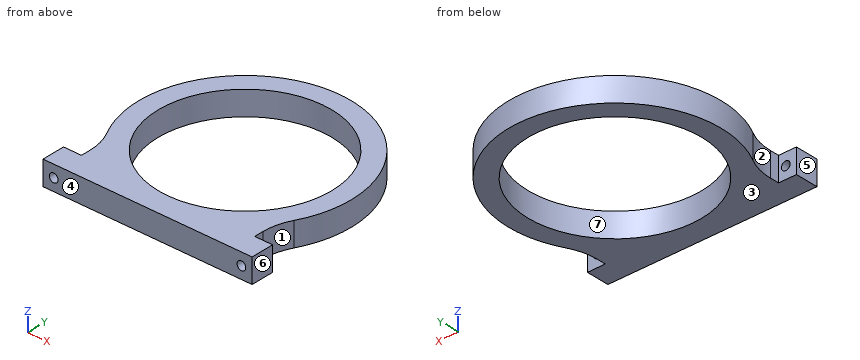
Autodesk Inventor part; units mm, degrees
ref_plane "YZ Plane" through (0, 0, 0) normal (1, 0, 0) x (0, 1, 0)
ref_plane "XZ Plane" through (0, 0, 0) normal (0, 1, 0) x (-1, 0, 0)
ref_plane "XY Plane" through (0, 0, 0) normal (0, 0, 1) x (1, 0, 0)
sketch "Sketch1" plane through (0, 0, 0) normal (0, 0, 1) x (1, 0, 0)
  line L0 (0, 0) -> (72.4, 0)
  line L1 (72.4, 0) -> (72.4, 8)
  line L2 (72.4, 8) -> (0, 8)
  line L3 (0, 8) -> (0, 0)
  line L4 (36.2, 8) -> (36.2, 38) construction
  circle A0 centre (36.2, 38) radius 30
  circle A1 centre (36.2, 38) radius 36.75
  line L5 (6.2, 8) -> (6.2, 16.7735)
  line L6 (66.2, 8) -> (66.2, 16.7735)
  dimension "d0" = 72.4
  dimension "d1" = 8
  dimension "d2" = 30
  dimension "d3" = 60
  dimension "d4" = 73.5
extrude "Extrusion1" add sketch "Sketch1" along normal blind 8.4
fillet "Fillet1" radius 20 2 edges at (66.2, 16.7735, 4.2) (6.2, 16.7735, 4.2)
sketch "Sketch2" plane through (0, 0, 0) normal (0, -1, 0) x (1, 0, 0)
  line L0 (72.4, 0) -> (72.4, 8.4)
  line L1 (0, 0) -> (0, 8.4) construction
  line L2 (0, 4.2) -> (3.7, 4.2) construction
  circle A0 centre (3.7, 4.2) radius 1.5
  line L3 (72.4, 4.2) -> (68.7, 4.2) construction
  circle A1 centre (68.7, 4.2) radius 1.5
  dimension "d8" = 3.7
  dimension "d9" = 3
  dimension "d10" = 3.7
  dimension "d11" = 3
extrude "Extrusion2" cut sketch "Sketch2" against normal up to surface (8 mm away)
properties part number "reservoir pump combo mount"
Can you work these out from the model? Positions are in its coordinate system, mm. Face numbers are marked on the shaded views. A direction names the side the tool comes from. Coordinates: 2 decimals unless noted, no trailing zeros. Loops run counter-clockwise (first coordinate to the right, second up) from the corner with the lowest first, then second, coordinate; pieces in that order, holes last. Notation, with made-up numbers: M 83.25,-28 L 99.25,-28 A29 ccw 99.25,-1 Z; hole C -27.75,33.5 d7. An arc over 180 degrees is marked long. Return JSON: item names as keys, results as strings. Group by question number.
Item 1: If I drill on L1, parallel to X at y = 38, z = 3.25; L2, parallel to Y at x = 10.5, z = 6.75; L3, parallel to Y at x = 29.5, z = 4.5, over which ranges is the centre line in solid material (lowest first)? Write a range as from..to.
Item 2: Imagine slicing it at B-B (y = 38). Please give me the cut outline in (x, z).
Item 3: Imagine slicing it at A-A (z = 4.2). Please give me the cut outline in (x, y).
Item 4: On a 3-axis mill with a long thin cutter (end or side, diameter ignored), from which of +Z, -Z, +X, -X, +Y, -Y can I reach the whole of each face in a straight line? I mean the marked faces 5, 6 and 7. Say none if no direction works.
Item 5: Imagine slicing it at C-C (x = 36.2). Please give me the cut outline in (y, z), and give its area (3 significant figures).
Item 6: I'm going to push flat-ended pins straight in: pin 1 Ø5 at (x, z) = (3.7, 4.2) entering from -Y; pin 2 Ø2 at (x, z) = (54, 2.5) entering from +Y; pin 3 Ø1.6 at (y, z) = (10.5, 5) entering from -X; pin 4 Ø1.9 at (x, z) = (69.5, 6) entering from +Y. Where does each tip first touch, or does it pass through?
Item 7: Thinking about a two-plate mould opening in Y: for the marked faces 1, 2, 3 and 4, which applies, released by +Y, released by -Y, zero draft, split by the parting line, or undercut?
Verdict:
{
 "1": {"L1": "x = -0.55..6.2, 66.2..72.95", "L2": "y = 0..22.52, 53.48..64.27", "L3": "y = 0..8.76, 67.24..74.13"},
 "2": {"outline": "M -0.55,0 L 6.2,0 L 6.2,8.4 L -0.55,8.4 Z; M 66.2,0 L 72.95,0 L 72.95,8.4 L 66.2,8.4 Z"},
 "3": {"outline": "M 0,0 L 2.2,0 L 2.2,8 L 0,8 Z; M 3.82,20.62 A20 cw 6.2,11.16 L 6.2,8 L 5.2,8 L 5.2,0 L 67.2,0 L 67.2,8 L 66.2,8 L 66.2,11.16 A20 cw 68.58,20.62 A36.75 ccw long Z; M 70.2,0 L 72.4,0 L 72.4,8 L 70.2,8 Z; hole C 36.2,38 d60"},
 "4": {"face 5": "+Z, -Z, -X, -Y", "face 6": "+Z, -Z, +X, -Y", "face 7": "+Z, -Z"},
 "5": {"outline": "M 0,0 L 8,0 L 8,8.4 L 0,8.4 Z; M 68,0 L 74.75,0 L 74.75,8.4 L 68,8.4 Z", "area": "124 mm^2"},
 "6": {"pin 1": "stops at y = 0", "pin 2": "stops at y = 70.69", "pin 3": "stops at x = 6.2", "pin 4": "stops at y = 55.44"},
 "7": {"face 1": "undercut", "face 2": "undercut", "face 3": "zero draft", "face 4": "released by -Y"}
}
